Check sheet for the modelled part. Datum: model origin and axes. Units: mm. A direction names the side the tool comes from. Give positions to 0.01 mm unless a question says otherwise; leave off trailing zeros. Order: outer loops, then holes, each group sorted by start corner. A loop starts at its lowest first (then second) coordinate and runs counter-clockwise, first axis right, second up. Notation, with made-up numbers: (70, -37.75) -> (100, -37.75) arc R12 ccw to (100, -27.75) -> close; hole circle Ø10 at (85, 19). An arc over 180 degrees is marked (long way). Write each question's results on one line, items separated by ' | '.
from build123d import *

# Parameters (mm, degrees)
SKETCH2_W           = 40
SKETCH2_H           = 6.6
BOSS_EXTRUDE1_DEPTH = 3
SKETCH3_W           = 35
SKETCH3_H           = 1.6
CUT_EXTRUDE1_DEPTH  = 1.5
BOSS_EXTRUDE2_DEPTH = 72
SKETCH5_W           = 22
SKETCH5_H           = 2.5
CUT_EXTRUDE2_DEPTH  = 4
SKETCH6_W           = 9
SKETCH6_H           = 3.25
BOSS_EXTRUDE3_DEPTH = 11
SKETCH7_W           = 9
SKETCH7_H           = 3.25
BOSS_EXTRUDE4_DEPTH = 11
SKETCH8_R           = 2
CUT_EXTRUDE3_DEPTH  = 3.25
FILLET1_R           = 2
FILLET2_R           = 5
FILLET3_R           = 5
FILLET4_R           = 2
FILLET5_R           = 5
FILLET6_R           = 5
FILLET7_R           = 2
FILLET8_R           = 2
FILLET9_R           = 5
FILLET10_R          = 5
FILLET11_R          = 5
FILLET12_R          = 5


with BuildPart() as part:
    # Sketch2 → Boss-Extrude1 (new body)
    with BuildSketch(Plane.XY):
        with Locations((-0.139783945, 0.84413532)):
            Rectangle(SKETCH2_W, SKETCH2_H)
    extrude(amount=BOSS_EXTRUDE1_DEPTH)

    # Sketch3 → Cut-Extrude1 (cut)
    with BuildSketch(Plane.XY.offset(3)):
        with Locations((-0.593876274, 0.84413532)):
            Rectangle(SKETCH3_W, SKETCH3_H)
    extrude(amount=-CUT_EXTRUDE1_DEPTH, mode=Mode.SUBTRACT)

    # Sketch4 → Boss-Extrude2 (add)
    with BuildSketch(Plane.XY.offset(3)):
        Polygon((-16.593876274, 4.14413532), (-20.139783945, 4.14413532), (-20.139783945, -2.45586468), (-16.593876274, -2.45586468), (-16.593876274, 0.04413532), (-18.093876274, 0.04413532), (-18.093876274, 1.64413532), (-16.593876274, 1.64413532), align=None)
        Polygon((15.406123726, 4.14413532), (15.406123726, 1.64413532), (16.906123726, 1.64413532), (16.906123726, 0.04413532), (15.406123726, 0.04413532), (15.406123726, -2.45586468), (19.860216055, -2.45586468), (19.860216055, 4.14413532), align=None)
    extrude(amount=BOSS_EXTRUDE2_DEPTH)

    # Sketch5 → Cut-Extrude2 (cut)
    with BuildSketch(Plane.XY.offset(3)):
        with Locations((4.406123726, -1.20586468)):
            Rectangle(SKETCH5_W, SKETCH5_H)
    extrude(amount=-CUT_EXTRUDE2_DEPTH, mode=Mode.SUBTRACT)

    # Sketch6 → Boss-Extrude3 (add)
    with BuildSketch(Plane.ZY.offset(20.139783945)):
        with Locations((19.5, -0.83086468)):
            Rectangle(SKETCH6_W, SKETCH6_H)
        with Locations((55.5, -0.83086468)):
            Rectangle(SKETCH6_W, SKETCH6_H)
    extrude(amount=BOSS_EXTRUDE3_DEPTH)

    # Sketch7 → Boss-Extrude4 (add)
    with BuildSketch(Plane(origin=(19.860216055, 0, 0), x_dir=(0, 0, -1), z_dir=(1, 0, 0))):
        with Locations((-55.5, -0.83086468)):
            Rectangle(SKETCH7_W, SKETCH7_H)
        with Locations((-19.5, -0.83086468)):
            Rectangle(SKETCH7_W, SKETCH7_H)
    extrude(amount=BOSS_EXTRUDE4_DEPTH)

    # Sketch8 → Cut-Extrude3 (cut)
    with BuildSketch(Plane(origin=(0, 0.79413532, 0), x_dir=(1, 0, 0), z_dir=(0, 1, 0))):
        with Locations((-26.639783945, -19.5)):
            Circle(SKETCH8_R)
        with Locations((-26.639783945, -55.5)):
            Circle(SKETCH8_R)
        with Locations((26.360216055, -55.5)):
            Circle(SKETCH8_R)
        with Locations((26.360216055, -19.5)):
            Circle(SKETCH8_R)
    extrude(amount=-CUT_EXTRUDE3_DEPTH, mode=Mode.SUBTRACT)

    # Fillet1
    fillet1_edges = [part.edges().sort_by_distance(p)[0] for p in [
        (19.860216055, 0.79413532, 55.5),
    ]]
    fillet(fillet1_edges, radius=FILLET1_R)

    # Fillet2
    fillet2_edges = [part.edges().sort_by_distance(p)[0] for p in [
        (19.860216055, -0.83086468, 51),
    ]]
    fillet(fillet2_edges, radius=FILLET2_R)

    # Fillet3
    fillet3_edges = [part.edges().sort_by_distance(p)[0] for p in [
        (19.860216055, -0.83086468, 60),
    ]]
    fillet(fillet3_edges, radius=FILLET3_R)

    # Fillet4
    fillet4_edges = [part.edges().sort_by_distance(p)[0] for p in [
        (19.860216055, 0.79413532, 19.5),
    ]]
    fillet(fillet4_edges, radius=FILLET4_R)

    # Fillet5
    fillet5_edges = [part.edges().sort_by_distance(p)[0] for p in [
        (19.860216055, -0.83086468, 15),
    ]]
    fillet(fillet5_edges, radius=FILLET5_R)

    # Fillet6
    fillet6_edges = [part.edges().sort_by_distance(p)[0] for p in [
        (19.860216055, -0.83086468, 24),
    ]]
    fillet(fillet6_edges, radius=FILLET6_R)

    # Fillet7
    fillet7_edges = [part.edges().sort_by_distance(p)[0] for p in [
        (-20.139783945, 0.79413532, 55.5),
    ]]
    fillet(fillet7_edges, radius=FILLET7_R)

    # Fillet8
    fillet8_edges = [part.edges().sort_by_distance(p)[0] for p in [
        (-20.139783945, 0.79413532, 19.5),
    ]]
    fillet(fillet8_edges, radius=FILLET8_R)

    # Fillet9
    fillet9_edges = [part.edges().sort_by_distance(p)[0] for p in [
        (-20.139783945, -0.83086468, 15),
    ]]
    fillet(fillet9_edges, radius=FILLET9_R)

    # Fillet10
    fillet10_edges = [part.edges().sort_by_distance(p)[0] for p in [
        (-20.139783945, -0.83086468, 24),
    ]]
    fillet(fillet10_edges, radius=FILLET10_R)

    # Fillet11
    fillet11_edges = [part.edges().sort_by_distance(p)[0] for p in [
        (-20.139783945, -0.83086468, 51),
    ]]
    fillet(fillet11_edges, radius=FILLET11_R)

    # Fillet12
    fillet12_edges = [part.edges().sort_by_distance(p)[0] for p in [
        (-20.139783945, -0.83086468, 60),
    ]]
    fillet(fillet12_edges, radius=FILLET12_R)


solid = part.part
1. Section check C-C on x = -15.5. Record the cut outline in (y, z).
Verdict:
outline: (-2.46, 0) -> (4.14, 0) -> (4.14, 3) -> (1.64, 3) -> (1.64, 1.5) -> (0.04, 1.5) -> (0.04, 3) -> (-2.46, 3) -> close
2. Access from +Z, -Z, +X, -X, +Y, -Y to the whole of each face (thin tool, end or side, straight path). Record for faces 1 (the flat face through (-28, -1, 60)), 2 (the flat face through (28, -1, 15)), 3 (the flat face through (-28, -1, 51)), 4 (the flat face through (-12, -1, 3)).
Verdict:
face 1: +Z, -X, +Y, -Y | face 2: -Z, +X, +Y, -Y | face 3: -X, +Y, -Y | face 4: +Z, +Y, -Y
3. Gauge pin test, flat ends, axial feed: pin 1 Ø2 at (y, z) = (-0.5, 35) entering from +X; pin 2 Ø3.5 at (x, y) = (28.5, -1.5) entering from -Z; pin 3 Ø2 at (y, z) = (2.5, 38.5) entering from -X; pin 4 Ø9 at (x, z) = (-9.5, 45) entering from +Y. Record the tip position at first contact, or that the pin passes through.
Verdict:
pin 1: stops at x = 19.86 | pin 2: stops at z = 15 | pin 3: stops at x = -20.14 | pin 4: passes through
4. Section check A-A on z = 37. Record the cut outline in (x, y).
Verdict:
outline: (-20.14, -2.46) -> (-16.59, -2.46) -> (-16.59, 0.04) -> (-18.09, 0.04) -> (-18.09, 1.64) -> (-16.59, 1.64) -> (-16.59, 4.14) -> (-20.14, 4.14) -> close; (15.41, -2.46) -> (19.86, -2.46) -> (19.86, 4.14) -> (15.41, 4.14) -> (15.41, 1.64) -> (16.91, 1.64) -> (16.91, 0.04) -> (15.41, 0.04) -> close
5. Mould release check, pull along X, two halves, no side actions. Record for faces 5 (the cylindrical face through (-21.57, -0.45, 61.5)), 6 (the flat face through (4, 0.044, 1)), 7 (the flat face through (-19.8, -2.456, 34.5)): +X half, -X half, draft (parallel to the pull), parting line (faces both ways), or undercut.
Verdict:
face 5: -X half | face 6: undercut | face 7: draft
6. Material ranges on probe 1 along X at (y, z) = (-0.3, 55.5); probe 2 along X at (y, z) = (-2, 35.5); probe 3 along Z at (x, y) = (-14.5, 0.5), recorded low to high. Write a range as from..to.
Verdict:
probe 1: x = -31.14..-28.64, -24.64..-16.59, 15.41..24.36, 28.36..30.86 | probe 2: x = -20.14..-16.59, 15.41..19.86 | probe 3: z = 0..1.5
7. Section check B-B on z = 55.5. Give the number of separate pieces and of enclosed holes in the cut face, then the cut area to 3 significant figures.
Verdict:
separate pieces: 4 | enclosed holes: 0 | area: 95.2 mm^2
